Read the model definition and answer for the solid it produces. Units are mm, in the model's axes. Face numbers are marked on the shaded views. A direction names the side the tool comes from. Give positions to 0.01 mm unless a question says otherwise; leave off trailing zeros. Write each loop counter-clockwise with the first axis right and the second up, starting at its lowest first coordinate (ties: lowest second). Pieces come first, ordered by that corner, then holes. Notation, with made-up numbers: (-20.75, -13) -> (-5.75, -13) arc R34 cw to (-5.75, 26) -> close; hole circle Ø8 at (70.5, 69.25). An arc over 180 degrees is marked (long way). Write item = value, one per line.
from build123d import *

# Parameters (mm, degrees)
F0_W           = 90
F0_H           = 90
F1_DEPTH       = 102.5
F6_D           = 48
F6_DEPTH       = 25
F6_TIP         = 14.4206548567
F8_DEPTH       = 45.001
F8_DEPTH_BACK  = 45.001
F9_R           = 10
F10_DEPTH      = 25
F10_DEPTH_BACK = 25
F12_D          = 10.5
F12_DEPTH      = 20
F12_TIP        = 3.1545182499
F14_D          = 3
F14_DEPTH      = 45
F14_TIP        = 0.9012909285
F15_D          = 14.5
F15_DEPTH      = 16
F15_TIP        = 4.3562394879


with BuildPart() as f1:
    # F0 (on Top) → F1 (new body)
    with BuildSketch(Plane.XY):
        Rectangle(F0_W, F0_H)
    extrude(amount=F1_DEPTH)

    # F3 (on 3pt) → F4 (revolve, cut)
    with BuildSketch(Plane(origin=(0, 0, 0), x_dir=(0.7071067812, 0.7071067812, 0), z_dir=(0.7071067812, -0.7071067812, 0))):
        with BuildLine():
            Line((-30, 102.5), (-63.6396103068, 102.5))
            Line((-63.6396103068, 102.5), (-63.6396103068, 47.5))
            Line((-63.6396103068, 47.5), (-31.6, 47.5))
            ThreePointArc((-31.6, 47.5), (-30.4686291501, 47.9686291501), (-30, 49.1))
            Line((-30, 49.1), (-30, 102.5))
        make_face()
        with BuildLine():
            Line((-63.6396103068, 17.5), (-63.6396103068, 0))
            Line((-63.6396103068, 0), (-30, 0))
            Line((-30, 0), (-30, 2.5))
            Line((-30, 2.5), (-28, 2.5))
            ThreePointArc((-28, 2.5), (-27.2928932188, 2.7928932188), (-27, 3.5))
            Line((-27, 3.5), (-27, 5.5))
            ThreePointArc((-27, 5.5), (-27.2928932188, 6.2071067812), (-28, 6.5))
            Line((-28, 6.5), (-30, 6.5))
            Line((-30, 6.5), (-30, 15.9))
            ThreePointArc((-30, 15.9), (-30.4686291501, 17.0313708499), (-31.6, 17.5))
            Line((-31.6, 17.5), (-63.6396103068, 17.5))
        make_face()
    revolve(axis=Axis((0, 0, 62.0171971386), (0, 0, 1)), mode=Mode.SUBTRACT)

    # F6
    with Locations(Plane(origin=(0, 0, 0), x_dir=(1, 0, 0), z_dir=(0, 0, -1))):
        with Locations((0, 0)):
            Hole(F6_D / 2, depth=F6_DEPTH)
            with Locations((0, 0, -(F6_DEPTH + F6_TIP / 2))):  # 118° drill point
                Cone(0, F6_D / 2, F6_TIP, mode=Mode.SUBTRACT)

    # F7 (on Front) → F8 (cut, two sides)
    with BuildSketch(Plane.XZ) as f8_sk:
        with BuildLine():
            Line((-45, 102.5), (-45, 47.5))
            Line((-45, 47.5), (-26.2, 47.5))
            ThreePointArc((-26.2, 47.5), (-25.3514718626, 47.8514718626), (-25, 48.7))
            Line((-25, 48.7), (-25, 102.5))
            Line((-25, 102.5), (-45, 102.5))
        make_face()
        with BuildLine():
            Line((-8.8, 47.5), (8.8, 47.5))
            ThreePointArc((8.8, 47.5), (9.6485281374, 47.8514718626), (10, 48.7))
            Line((10, 48.7), (10, 102.5))
            Line((10, 102.5), (-10, 102.5))
            Line((-10, 102.5), (-10, 48.7))
            ThreePointArc((-10, 48.7), (-9.6485281374, 47.8514718626), (-8.8, 47.5))
        make_face()
        with BuildLine():
            Line((26.2, 47.5), (45, 47.5))
            Line((45, 47.5), (45, 102.5))
            Line((45, 102.5), (25, 102.5))
            Line((25, 102.5), (25, 48.7))
            ThreePointArc((25, 48.7), (25.3514718626, 47.8514718626), (26.2, 47.5))
        make_face()
    extrude(amount=-F8_DEPTH, mode=Mode.SUBTRACT)
    extrude(f8_sk.sketch, amount=F8_DEPTH_BACK, mode=Mode.SUBTRACT)

    # F9 (on Right) → F10 (cut, two sides)
    with BuildSketch(Plane.YZ) as f10_sk:
        with BuildLine():
            ThreePointArc((-28.2842712475, 82.5), (-17.3205080757, 96.9948974278), (0, 102.5))
            Line((0, 102.5), (-28.2842712475, 102.5))
            Line((-28.2842712475, 102.5), (-28.2842712475, 82.5))
        make_face()
        with BuildLine():
            ThreePointArc((0, 102.5), (17.3205080757, 96.9948974278), (28.2842712475, 82.5))
            Line((28.2842712475, 82.5), (28.2842712475, 102.5))
            Line((28.2842712475, 102.5), (0, 102.5))
        make_face()
        with Locations((0, 77.5)):
            Circle(F9_R)
    extrude(amount=-F10_DEPTH, mode=Mode.SUBTRACT)
    extrude(f10_sk.sketch, amount=F10_DEPTH_BACK, mode=Mode.SUBTRACT)

    # F12
    with Locations(Plane(origin=(0, 0, 17.5), x_dir=(1, 0, 0), z_dir=(0, 0, -1))):
        with Locations((-31.8198051534, -31.8198051534), (-31.8198051534, 31.8198051534), (31.8198051534, 31.8198051534), (31.8198051534, -31.8198051534)):
            Hole(F12_D / 2, depth=F12_DEPTH)
            with Locations((0, 0, -(F12_DEPTH + F12_TIP / 2))):  # 118° drill point
                Cone(0, F12_D / 2, F12_TIP, mode=Mode.SUBTRACT)

    # F14
    with Locations(Plane.XZ.offset(45)):
        with Locations((0, 32.5)):
            Hole(F14_D / 2, depth=F14_DEPTH)
            with Locations((0, 0, -(F14_DEPTH + F14_TIP / 2))):  # 118° drill point
                Cone(0, F14_D / 2, F14_TIP, mode=Mode.SUBTRACT)

    # F15
    with Locations(Plane.XZ.offset(45)):
        with Locations((0, 32.5)):
            Hole(F15_D / 2, depth=F15_DEPTH)
            with Locations((0, 0, -(F15_DEPTH + F15_TIP / 2))):  # 118° drill point
                Cone(0, F15_D / 2, F15_TIP, mode=Mode.SUBTRACT)


solid = f1.part
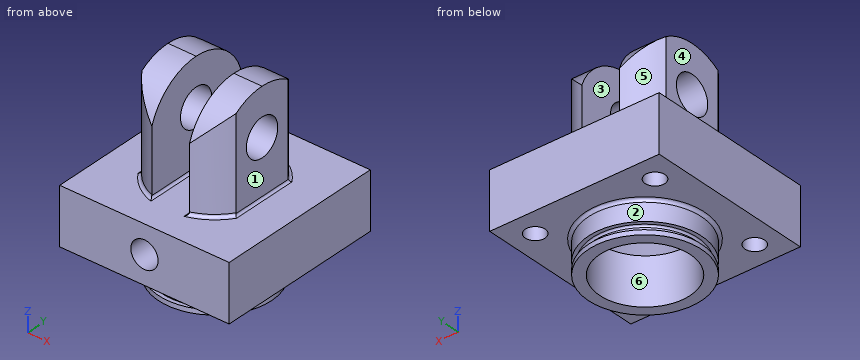
(1) The part is cut by section B-B on z = 77.5. Determine the outline of the cut face in (x, y), plus the area to 3 significant figures.
Checks:
outline = (-25, -16.58) arc R30 ccw to (-10, -28.28) -> (-10, -10) -> (-25, -10) -> close; (-25, 10) -> (-10, 10) -> (-10, 28.28) arc R30 ccw to (-25, 16.58) -> close; (10, -28.28) arc R30 ccw to (25, -16.58) -> (25, -10) -> (10, -10) -> close; (10, 10) -> (25, 10) -> (25, 16.58) arc R30 ccw to (10, 28.28) -> close
area = 825 mm²
(2) The part is cut by section C-C on y = 2. Count the separate pieces of the cut face and the enclosed holes in it, plus the area to 3 significant figures.
Checks:
separate_pieces = 3
enclosed_holes = 0
area = 3,250 mm²
(3) Given P1, Ø10, axis at y = -3, z = 76, coming from the -X side; P2, Ø4, axis at x = -17.5, y = 13.5, coming from the +Z side; P3, Ø17, axis at x = -31.82, y = 31.82, coming from the +Z side; P4, Ø2, axis at x = -25, y = 17, coming from the +Z side, each flat-ended and moving along its own axis, determine where each tip first touches the part or whether it passes through.
Checks:
P1 = through
P2 = 100.21
P3 = 47.5
P4 = 97.88
(4) The part is cut by section D-D on z = 21. Determine the outline of the cut face in (x, y), plus the area to 3 significant figures.
Checks:
outline = (-45, -45) -> (45, -45) -> (45, 45) -> (-45, 45) -> close; hole circle Ø10.5 at (-31.82, -31.82); hole circle Ø10.5 at (-31.82, 31.82); hole circle Ø48 at (0, 0); hole circle Ø10.5 at (31.82, -31.82); hole circle Ø10.5 at (31.82, 31.82)
area = 5,940 mm²
(5) For a pull along Y with two mould halves and no side action, classify the marked faces 4, 5 and 6 as released by +Y, released by -Y, zero draft, split by the parting line, or undercut.
Checks:
face_4 = zero draft
face_5 = released by +Y
face_6 = undercut
(6) Consider L1, parallel to X at y = -12.5, z = 97.5; L2, parallel to X at y = -14.5, z = 32.5; L3, parallel to Z at x = 21.5, y = 1. Determine where each line is inside the solid, lowest interval first.
Checks:
L1 = -25 to -10, 10 to 25
L2 = -45 to -1.5, 1.5 to 45
L3 = 26.49 to 67.55, 87.45 to 102.48
(7) The part is cut by section A-A on z = 56. Determine the outline of the cut face in (x, y), plus the area to 3 significant figures.
Checks:
outline = (-25, -16.58) arc R30 ccw to (-10, -28.28) -> (-10, 28.28) arc R30 ccw to (-25, 16.58) -> close; (10, -28.28) arc R30 ccw to (25, -16.58) -> (25, 16.58) arc R30 ccw to (10, 28.28) -> close
area = 1,420 mm²
(8) A tool of negligible diameter and unlimited length cuts with its end or side. For the marked faces 1, 2 and 3, from which of +Z, -Z, +X, -X, +Y, -Y can it reach the whole face along a straight path? Write none if from no direction.
Checks:
face_1 = +Z, +X, +Y, -Y
face_2 = -Z
face_3 = +Z, +Y, -Y
